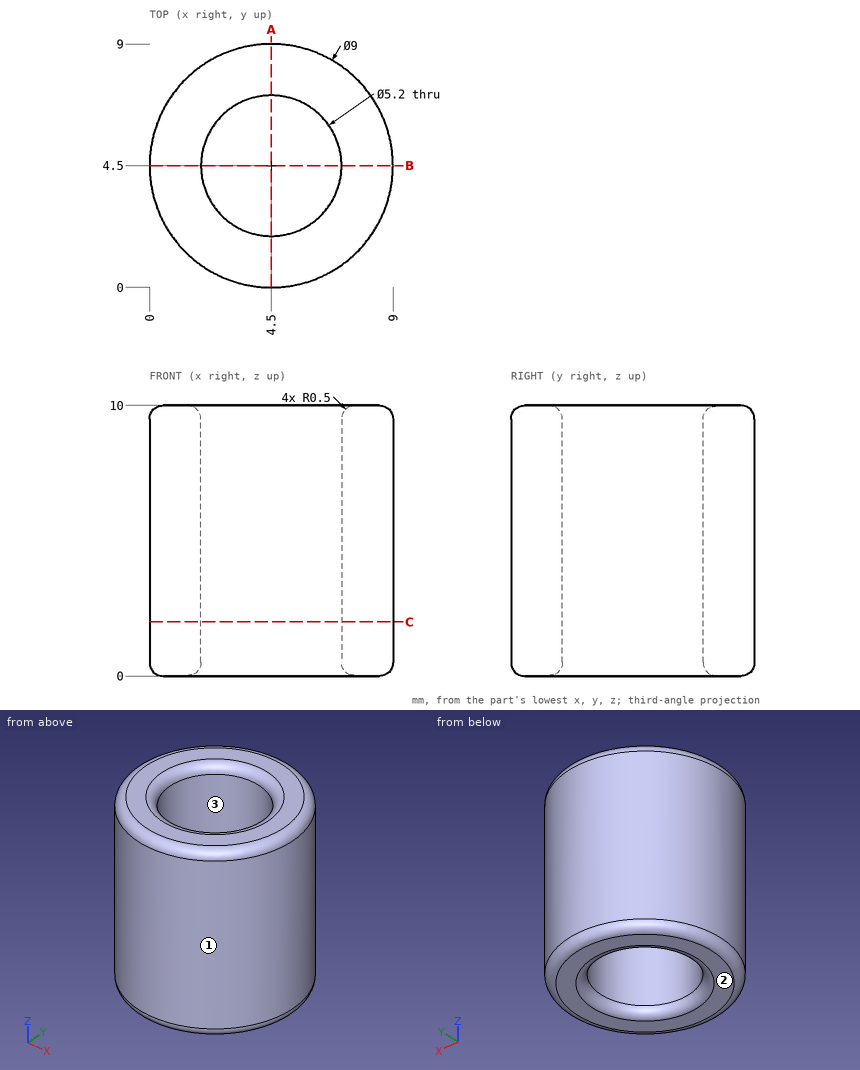
Study the drawing (mm; zero at the part's minimum x, y, z) and answer. Round coordinates to 2 decimals unless told otherwise and drop trailing zeros. Loops run counter-clockwise (first coordinate to the right, second up) from the corner with the lowest first, then second, coordinate; pieces in that order, holes last. Notation, with made-up numbers: (21.25, 87.25) -> (36.25, 87.25) arc R25 ccw to (36.25, 115.25) -> close; hole circle Ø4 at (-14.5, 69). An arc over 180 degrees is marked (long way). Use one line per item in the form item = value.
1. The part is cut by section A-A on x = 4.5. Determine the outline of the cut face in (y, z), and give its area (3 significant figures).
Answer key:
outline = (0, 0.5) arc R0.5 ccw to (0.5, 0) -> (1.4, 0) arc R0.5 ccw to (1.9, 0.5) -> (1.9, 9.5) arc R0.5 ccw to (1.4, 10) -> (0.5, 10) arc R0.5 ccw to (0, 9.5) -> close; (7.1, 0.5) arc R0.5 ccw to (7.6, 0) -> (8.5, 0) arc R0.5 ccw to (9, 0.5) -> (9, 9.5) arc R0.5 ccw to (8.5, 10) -> (7.6, 10) arc R0.5 ccw to (7.1, 9.5) -> close
area = 37.6 mm²
2. For a pull along Y with two mould halves and no side action, classify the marked faces 1, 2 and 3 as released by +Y, released by -Y, zero draft, split by the parting line, or undercut.
Answer key:
face_1 = split by the parting line
face_2 = zero draft
face_3 = undercut
3. The part is cut by section C-C on z = 2. Determine the outline of the cut face in (x, y), and give its area (3 significant figures).
Answer key:
outline = circle Ø9 at (4.5, 4.5); hole circle Ø5.2 at (4.5, 4.5)
area = 42.4 mm²
4. Find the intervals of material crossed by probe 1 along Y at (x, z) = (4.5, 6); probe 2 along Y at (x, z) = (5.5, 5); probe 3 along X at (y, z) = (4, 9.25), in increasing order. Write a range as [from, to].
Answer key:
probe_1 = [0, 1.9], [7.1, 9]
probe_2 = [0.11, 2.1], [6.9, 8.89]
probe_3 = [0.03, 1.95], [7.05, 8.97]
